Read the model definition and answer for the solid it produces. Units are mm, in the model's axes. Face numbers are marked on the shaded views. A direction names the side the tool comes from. Round coordinates to 2 decimals unless told otherwise and drop trailing zeros. Order: outer loops, then holes, each group sorted by start corner. A loop starts at its lowest first (then second) coordinate and runs counter-clockwise, first axis right, second up. Notation, with made-up numbers: (19, -31) - (72, -31) arc R11 ccw to (72, -27) - close; hole circle Ø7 at (-12, 70). An arc over 180 degrees is marked (long way). Answer as a JSON object with one key per item and string values. Group by question number.
Q1. A cutting plane is placed at D-D on y = -7.2. Determine the outline of the cut face in (x, z).
Q2. A tool of negligible diameter and unlimited length cuts with its end or side. For the marked faces 5, 6, 7, 8 and 9, from which of +Z, -Z, +X, -X, +Y, -Y can it reach the whole face along a straight path? Write none if from no direction.
Q3. A cutting plane is placed at C-C on z = -1. Determine the outline of the cut face in (x, y).
Q4. The mould has two halves that part along Z. Classify the marked faces 1, 2, 3 and 4: pulls with the +Z half, pulls with the -Z half, needs draft (parallel to the pull), parting line crosses it, or undercut.
Q5. A cutting plane is placed at A-A on x = 0. Determine the outline of the cut face in (y, z), and give its area (3 significant figures).
Q6. Consider line 1 (X direction, y = -5, z = 1.5); line 2 (Y direction, x = 0, z = -3.8); line 3 (Z direction, x = -14.25, y = -7.2). Determine where each line is inside the solid, lowest interval first.
Q7. Given pin 1 Ø11 at (x, y) = (-1.5, 7.5) entering from +Z; pin 2 Ø2 at (x, z) = (8.5, 1) entering from -Y; pin 3 Ø5 at (x, z) = (-3.5, 3.5) entering from +Y, each flat-ended and moving along its own axis, determine where each tip first touches the part or whether it passes through.
Q8. A cutting plane is placed at B-B on y = 7.5. Determine the outline of the cut face in (x, z).
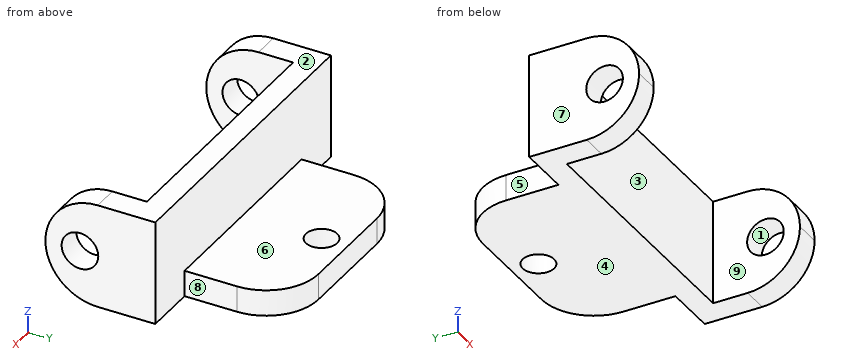
```python
from build123d import *

# Parameters (mm, degrees)
F0_W      = 25
F0_H      = 10
F1_DEPTH  = 2.2
F0_W_2    = 2.5
F2_DEPTH  = 10.5
F3_R      = 4.99999
F4_R      = 1.75
F5_DEPTH  = 35
F6_W      = 20
F6_H      = 2.5
F7_DEPTH  = 10
F8_R      = 5
F9_R      = 1.5
F10_DEPTH = 25


# Not quite as in the source:
# - a fillet or chamfer is up to 0.001 mm smaller than in the source, because OpenCascade refuses the exact size


with BuildPart() as f1:
    # F0 (on Front) → F1 (new body)
    with BuildSketch(Plane.XZ):
        Rectangle(F0_W, F0_H)
    extrude(amount=F1_DEPTH)

    # F0 (on Front) → F2 (join)
    with BuildSketch(Plane.XZ):
        with Locations((-13.75, 0)):
            Rectangle(F0_W_2, F0_H)
        with Locations((13.75, 0)):
            Rectangle(F0_W_2, F0_H)
    extrude(amount=F2_DEPTH)

    # F3 (radius 5 in the source; OpenCascade refuses exactly that, so slightly less here)
    f3_edges = [f1.edges().sort_by_distance(p)[0] for p in [
        (13.75, -10.5, 5),
        (13.75, -10.5, -5),
        (-13.75, -10.5, -5),
        (-13.75, -10.5, 5),
    ]]
    fillet(f3_edges, radius=F3_R)

    # F4 (on face) → F5 (cut)
    with BuildSketch(Plane.YZ.offset(15)):
        with Locations((-7.2, 0)):
            Circle(F4_R)
    extrude(amount=-F5_DEPTH, mode=Mode.SUBTRACT)

    # F6 (on face) → F7 (join)
    with BuildSketch(Plane(origin=(0, 0, 0), x_dir=(-1, 0, 0), z_dir=(0, 1, 0))):
        with Locations((0, -3.75)):
            Rectangle(F6_W, F6_H)
    extrude(amount=F7_DEPTH)

    # F8
    f8_edges = [f1.edges().sort_by_distance(p)[0] for p in [
        (10, 10, -3.75),
        (-10, 10, -3.75),
    ]]
    fillet(f8_edges, radius=F8_R)

    # F9 (on face) → F10 (cut)
    with BuildSketch(Plane(origin=(0, 0, -5), x_dir=(1, 0, 0), z_dir=(0, 0, -1))):
        with Locations((0, -7.5)):
            Circle(F9_R)
    extrude(amount=-F10_DEPTH, mode=Mode.SUBTRACT)


solid = f1.part
```
Result set:
{
 "1": {"outline": "(-15, -4.7) - (-12.5, -4.7) - (-12.5, -1.75) - (-15, -1.75) - close; (-15, 1.75) - (-12.5, 1.75) - (-12.5, 4.7) - (-15, 4.7) - close; (12.5, -4.7) - (15, -4.7) - (15, -1.75) - (12.5, -1.75) - close; (12.5, 1.75) - (15, 1.75) - (15, 4.7) - (12.5, 4.7) - close"},
 "2": {"face 5": "+Z, -Z, -X, +Y", "face 6": "+Z, +X, -X, +Y", "face 7": "+Z, -Z, -X, +Y, -Y", "face 8": "+Z, -Z, +X, +Y", "face 9": "+Z, -Z, -Y"},
 "3": {"outline": "(-15, -10.4) - (-12.5, -10.4) - (-12.5, -8.64) - (-15, -8.64) - close; (-15, -5.76) - (-12.5, -5.76) - (-12.5, -2.2) - (12.5, -2.2) - (12.5, -5.76) - (15, -5.76) - (15, 0) - (-15, 0) - close; (12.5, -10.4) - (15, -10.4) - (15, -8.64) - (12.5, -8.64) - close"},
 "4": {"face 1": "undercut", "face 2": "pulls with the +Z half", "face 3": "needs draft", "face 4": "pulls with the -Z half"},
 "5": {"outline": "(-2.2, -5) - (6, -5) - (6, -2.5) - (0, -2.5) - (0, 5) - (-2.2, 5) - close; (9, -5) - (10, -5) - (10, -2.5) - (9, -2.5) - close", "area": "39.5 mm²"},
 "6": {"line 1": "x = -15 to -12.5, 12.5 to 15", "line 2": "y = -2.2 to 6, 9 to 10", "line 3": "z = -4.7 to -1.75, 1.75 to 4.7"},
 "7": {"pin 1": "stops at z = -2.5", "pin 2": "stops at y = -2.2", "pin 3": "stops at y = 0"},
 "8": {"outline": "(-9.33, -5) - (-1.5, -5) - (-1.5, -2.5) - (-9.33, -2.5) - close; (1.5, -5) - (9.33, -5) - (9.33, -2.5) - (1.5, -2.5) - close"}
}
